```python
from build123d import *

# Parameters (mm, degrees)
F3_DEPTH = 3.05
F4_R     = 1.425
F5_DEPTH = 20


with BuildPart() as f1:
    # F0 (on Front) → F1 (revolve)
    with BuildSketch(Plane.XZ):
        Polygon((0, 9.5), (0, 0), (73, 0), (73, 3.175), (69.92, 3.175), (69.92, 4.955), (52.92, 5.5), (45, 6), (2, 6.885), (2, 9.5), align=None)
    revolve(axis=Axis((36.5, 0, 0), (1, 0, 0)))

    # F2 (on face) → F3 (join)
    with BuildSketch(Plane.YZ.offset(69.92)):
        with BuildLine():
            Line((4.61, -0.85), (4.61, 0.85))
            Line((4.61, 0.85), (3.059105, 0.85))
            ThreePointArc((3.059105, 0.85), (3.145893, 0.428932), (3.175, 0))
            ThreePointArc((3.175, 0), (3.145893, -0.428932), (3.059105, -0.85))
            Line((3.059105, -0.85), (4.61, -0.85))
        make_face()
        with BuildLine():
            ThreePointArc((3.175, 0), (3.145893, 0.428932), (3.059105, 0.85))
            ThreePointArc((3.059105, 0.85), (-3.175, 0), (3.059105, -0.85))
            ThreePointArc((3.059105, -0.85), (3.145893, -0.428932), (3.175, 0))
        make_face()
    extrude(amount=F3_DEPTH)

    # F4 (on face) → F5 (cut)
    with BuildSketch(Plane.YZ.offset(73)):
        Circle(F4_R)
    extrude(amount=-F5_DEPTH, mode=Mode.SUBTRACT)


solid = f1.part
```
Geometry check sheet. Reference: the model listing, model coordinates, mm. A direction names the side the tool comes from. Coordinates: 2 decimals unless noted, no trailing zeros. Order: outer loops, then holes, each group sorted by start corner. A loop starts at its lowest first (then second) coordinate and runs counter-clockwise, first axis right, second up. Notation, with made-up numbers: (-35, -26) - (15, -26) arc R14 cw to (15, -3) - close; hole circle Ø11 at (43.25, 61). An arc over 180 degrees is marked (long way). Answer in a Markdown table with one row per item. Add a question column.
1. Section check D-D (x = 13). Enter the section's corners in (y, z).
2. Section check C-C (x = 65). Enter the section's corners in (y, z) (3 decimals).
3. Draft check along Y on faces 1 (the face through (53, 0, 0)), 2 (the face through (69.92, -3.4, 0.1)), 3 (the face through (61.3, -1.57, 4.99)). Enter one of: +Y half, -Y half, draft (parallel to the pull), parting line (faces both ways), or undercut.
4. Access from +Z, -Z, +X, -X, +Y, -Y to the whole of each face (thin tool, end or side, straight path). Record for faces 4 (the face through (71, 4, -0.85)), 5 (the face through (71, 4, 0.85)), 6 (the face through (0.99, 8.43, 4.38)), 7 (the face through (71, 4.61, 0)), 8 (the face through (2, -5, -5)).
5. Material ranges on L1, parallel to X at y = -6.25, z = -4.5; L2, parallel to Z at x = 60.5, y = 0 (3 decimals); L3, parallel to X at y = 0.75, z = -3.5, recorded low to high. Write a range as [from, to].
6. Section check A-A (y = 0). Enter the section's corners in (x, z) (3 decimals).
7. Gauge pin test, flat ends, axial feed: pin 1 Ø2.5 at (y, z) = (0, 0) entering from +X; pin 2 Ø0.8 at (y, z) = (4, 0) entering from +X; pin 3 Ø1.2 at (x, y) = (72, 4) entering from +Z. Record the tip position at first contact, or that the pin passes through.
8. Section check B-B (z = 0). Enter the section's corners in (x, y) (3 decimals).
Data:
| question | item | result |
|---|---|---|
| 1 | outline | circle Ø13.32 at (0, 0) |
| 2 | outline | circle Ø10.225 at (0, 0); hole circle Ø2.85 at (0, 0) |
| 3 | face 1 | undercut |
| 3 | face 2 | draft |
| 3 | face 3 | parting line |
| 4 | face 4 | -Z, +X, +Y |
| 4 | face 5 | +Z, +X, +Y |
| 4 | face 6 | +X, -X |
| 4 | face 7 | +Z, -Z, +X, +Y |
| 4 | face 8 | +X |
| 5 | L1 | x = [0, 2] |
| 5 | L2 | z = [-5.257, -1.425], [1.425, 5.257] |
| 5 | L3 | x = [0, 69.92] |
| 6 | outline | (0, -9.5) - (2, -9.5) - (2, -6.885) - (45, -6) - (52.92, -5.5) - (69.92, -4.955) - (69.92, -3.175) - (73, -3.175) - (73, -1.425) - (53, -1.425) - (53, 1.425) - (73, 1.425) - (73, 3.175) - (69.92, 3.175) - (69.92, 4.955) - (52.92, 5.5) - (45, 6) - (2, 6.885) - (2, 9.5) - (0, 9.5) - close |
| 7 | pin 1 | stops at x = 53 |
| 7 | pin 2 | stops at x = 72.97 |
| 7 | pin 3 | stops at z = 0.85 |
| 8 | outline | (0, -9.5) - (2, -9.5) - (2, -6.885) - (45, -6) - (52.92, -5.5) - (69.92, -4.955) - (69.92, -3.175) - (73, -3.175) - (73, -1.425) - (53, -1.425) - (53, 1.425) - (73, 1.425) - (73, 3.175) - (72.97, 3.175) - (72.97, 4.61) - (69.92, 4.61) - (69.92, 4.955) - (52.92, 5.5) - (45, 6) - (2, 6.885) - (2, 9.5) - (0, 9.5) - close |
